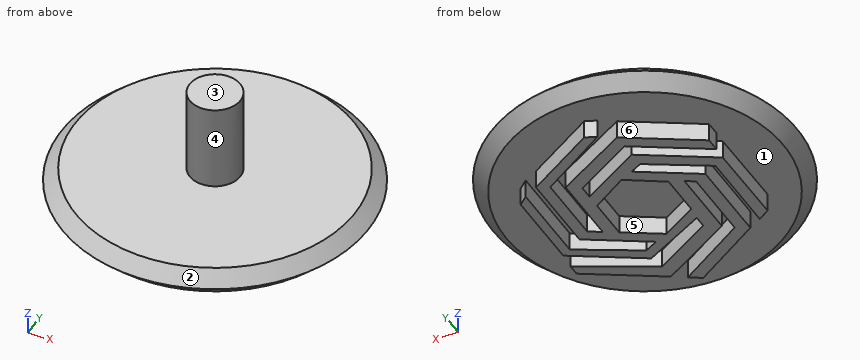
from build123d import *

# Parameters (mm, degrees)
F0_R     = 19.05
F1_DEPTH = 3.302
F2_R     = 3.0940455734
F3_DEPTH = 10.668
F4_SIZE  = 2.032
F7_DEPTH = 2.286


# Not quite as in the source:
# - a fillet or chamfer that OpenCascade refuses, or shapes differently, is made with other operations: its cross-section is extruded or revolved along the edge and cut away or added


with BuildPart() as f1:
    # F0 (on Top) → F1 (new body)
    with BuildSketch(Plane.XY):
        Circle(F0_R)
    extrude(amount=F1_DEPTH)

    # F2 (on face) → F3 (join)
    with BuildSketch(Plane.XY.offset(3.302)):
        Circle(F2_R)
    extrude(amount=F3_DEPTH)

    # F4
    f4_edges = [f1.edges().sort_by_distance(p)[0] for p in [
        (-19.05, 0, 3.302),
    ]]
    chamfer(f4_edges, length=F4_SIZE)

    # F5: chamfer of 2.032 on 1 edges, made by hand

    # F5_s1 → F5_t2 (revolve, cut)
    with BuildSketch(Plane.XZ):
        Polygon((19.05, 2.032), (17.018, 0), (19.05, 0), align=None)
    revolve(axis=Axis((0, 0, 0), (0, 0, 1)), mode=Mode.SUBTRACT)

    # F6 (on face) → F7 (join)
    with BuildSketch(Plane(origin=(0, 0, 0), x_dir=(1, 0, 0), z_dir=(0, 0, -1))):
        Polygon((-10.1241571829, 7.50669837), (-11.5505903959, 6.6151777282), (-11.4901715756, -3.6598756731), (-2.9577685054, -8.7351842692), (4.4179176912, -4.5286850072), (4.4179176912, -6.1632911675), (-2.9577685054, -10.3697904294), (-11.5558920335, -5.255389493), (-11.5558920335, -6.9493146705), (-2.9577685054, -12.0637156069), (5.9589991364, -7.1465903893), (5.9589991364, 1.4732169604), (7.414681837, 0.6073367549), (7.414681837, -7.955128327), (-1.1376237962, -13.150122948), (0.1876302122, -13.7365777045), (8.8004540583, -8.6443684995), (8.8004540583, 1.404343208), (1.6391712, 5.6640716984), (3.2676828559, 6.4783277921), (10.5352541432, 2.4422151037), (10.5352541432, -7.7702743001), (11.6456285548, -6.8170730956), (11.6456285548, 3.0340532394), (3.4269623458, 7.9227425003), (-4.1806832887, 4.1189184412), (-4.1806832887, 5.604787264), (3.0703544617, 9.7057837993), (11.8158220797, 5.0698746927), (11.8158220797, 6.4297318659), (3.0109197833, 11.667130515), (-5.9344387757, 6.6151777282), (-5.9344387757, -2.0622941665), (-7.0335506462, -1.408512122), (-7.0335506462, 7.50669837), (1.4481722892, 12.6481941369), (0, 13.5096069425), (-8.5194194689, 8.338784799), (-8.5194194689, -2.0622941665), (-1.6249895561, -6.1632911675), (-3.0514232349, -6.8765082397), (-10.1241571829, -2.7755110059), align=None)
        Polygon((0, -5.4471737376), (-4.3624499813, -2.7635633014), (-4.3624499813, 2.5107886177), (0, 4.998779855), (4.4179176912, 2.3708806043), (4.4179176912, -2.7635630686), align=None, mode=Mode.SUBTRACT)
    extrude(amount=F7_DEPTH)


solid = f1.part
Could you check a few things on this model? Use its own coordinates, in mm. Face numbers are marked on the shaded views. A direction names the side the tool comes from. Coordinates: 2 decimals unless noted, no trailing zeros. Loops run counter-clockwise (first coordinate to the right, second up) from the corner with the lowest first, then second, coordinate; pieces in that order, holes last.
1. Imagine slicing it at B-B (z = 11.25). Please give me the cut outline in (x, y).
2. For P1, Ø6, axis at y = -11.5, z = -0.5, coming from the +X side; P2, Ø1.1, axis at y = -1, z = -1, coming from the +X side; P3, Ø4, axis at x = 0, y = 6, coming from the +Z side; P4, Ø5, axis at y = -6.5, z = 10, coming from the -X side, each with a flat end and sliding along its axis, tell me the tip position at first contact or that it passes through.
3. For the marked faces 4, 5 and 6, which set-ups out of +Z, -Z, +X, -X, +Y, -Y let a thin tool reach every point of the face, with its end or its side?
4. We'd pull the mould along X, two halves only. Please class the marked faces 1, 2 and 3: released by +X, released by -X, zero draft, split by the parting line, or undercut.
5. Imagine slicing it at C-C (z = 2.75). Please give me the cut outline in (x, y).
6. I need wall thicknesses on L1, parallel to Z at x = 1.5, y = -4; L2, parallel to Z at x = 2, y = 5.5; L3, parallel to Y at x = -11, z = -1.5. Which ranges of each line are inside material? Lowest first, please.
Computed values:
1. outline: circle Ø6.19 at (0, 0)
2. P1: stops at x = 16.12
2. P2: stops at x = 11.65
2. P3: stops at z = 3.3
2. P4: passes through
3. face 4: +Z
3. face 5: -Z
3. face 6: -Z, -X, +Y
4. face 1: undercut
4. face 2: split by the parting line
4. face 3: zero draft
5. outline: circle Ø35.14 at (0, 0)
6. L1: z = 0 to 3.3
6. L2: z = -2.29 to 3.3
6. L3: y = -6.96 to 3.95, 5.59 to 7.28
